from build123d import *

# Parameters (mm, degrees)
F0_W          = 812.8
F0_H          = 101.6
F1_DEPTH      = 482.6
F2_W          = 812.8
F2_H          = 228.6
F3_DEPTH      = 734.06
F3_DEPTH_BACK = 482.6
F4_W          = 812.8
F4_H          = 596.9
F5_DEPTH      = 1219.2
F6_W          = 812.8
F6_H          = 1397
F7_DEPTH      = 762
F8_W          = 657.52998
F8_H          = 629.62246
F9_DEPTH      = 774.7


with BuildPart() as f1:
    # F0 (on Top) → F1 (new body)
    with BuildSketch(Plane.XY):
        with Locations((406.4, 50.8)):
            Rectangle(F0_W, F0_H)
    extrude(amount=F1_DEPTH)

    # F2 (on face) → F3 (join, two sides)
    with BuildSketch(Plane.XY.offset(482.6)) as f3_sk:
        with Locations((406.4, 215.9)):
            Rectangle(F2_W, F2_H)
    extrude(amount=F3_DEPTH)
    extrude(f3_sk.sketch, amount=-F3_DEPTH_BACK)

    # F4 (on Top) → F5 (join)
    with BuildSketch(Plane.XY):
        with Locations((406.4, 628.65)):
            Rectangle(F4_W, F4_H)
    extrude(amount=F5_DEPTH)

    # F6 (on face) → F7 (join)
    with BuildSketch(Plane(origin=(0, 927.1, 0), x_dir=(-1, 0, 0), z_dir=(0, 1, 0))):
        with Locations((-406.4, 698.5)):
            Rectangle(F6_W, F6_H)
    extrude(amount=F7_DEPTH)

    # F8 (on face) → F9 (cut)
    with BuildSketch(Plane.XY.offset(1397)):
        with Locations((423.118338, 1320.792675)):
            Rectangle(F8_W, F8_H)
    extrude(amount=-F9_DEPTH, mode=Mode.SUBTRACT)


solid = f1.part
CAD build for the part. Positions are in the model's coordinates, mm. A direction names the side the tool comes from. Coordinates: 2 decimals unless noted, no trailing zeros. Loops run counter-clockwise (first coordinate to the right, second up) from the corner with the lowest first, then second, coordinate; pieces in that order, holes last. Notation, with made-up numbers: (80.5, -27.5) - (94.5, -27.5) arc R8 ccw to (94.5, -20.5) - close; hole circle Ø6 at (43, -14.75). An arc over 180 degrees is marked (long way). Use one line per item in the form item = value. Start each with the question number.
1) Band-saw the part on A-A (z = 872). Give the cut face in (x, y), and give its area (3 significant figures).
2) Drill centre lines: L1, parallel to X at y = 1047, z = 785; L2, parallel to Y at x = 287.5, z = 716; L3, parallel to Y at x = 432.5, z = 1288.5. Where is each one in solid material? Low to high. Write a range as from..to.
3) Band-saw the part on B-B (x = 318). Give the cut face in (y, z), and give its area (3 significant figures).
4) Tool access for faces 1 (the face through (419, 1005.981, 1015)), 2 (the face through (812.8, 833, 689)), 3 (the face through (401, 52, 482.6)): list every direction of +Z, -Z, +X, -X, +Y, -Y with a clear straight run to the whole face (end or side of a thin tool).
5) Flat gauge pins, fed straight in: pin 1 (2 mm diameter, centred on x = 215.5, z = 502.5, fed in from -Y); pin 2 (1.3 mm diameter, centred on x = 557.5, z = 1217.5, fed in from -Y). Where does each tip first touch, or does it go through?
6) Band-saw the part on C-C (y = 895). Give the cut face in (x, z), and give its area (3 significant figures).
7) Band-saw the part on D-D (y = 229). Give the cut face in (x, z), and give its area (3 significant figures).
8) Two-plate mould, pull along X, no slides. Class faces 4 (the face through (401, 101.6, 844)), 5 (the face through (0, 833, 689)), 6 (the face through (751.883, 1316, 1015)): +X half, -X half, draft (parallel to the pull), parting line (faces both ways), or undercut.
Check values:
q1.outline = (0, 101.6) - (812.8, 101.6) - (812.8, 1689.1) - (0, 1689.1) - close; hole (94.35, 1005.98) - (751.88, 1005.98) - (751.88, 1635.6) - (94.35, 1635.6) - close
q1.area = 876,000 mm2
q2.L1 = 0..94.35, 751.88..812.8
q2.L2 = 101.6..1005.98, 1635.6..1689.1
q2.L3 = 927.1..1005.98, 1635.6..1689.1
q3.outline = (0, 0) - (1689.1, 0) - (1689.1, 1397) - (1635.6, 1397) - (1635.6, 622.3) - (1005.98, 622.3) - (1005.98, 1397) - (927.1, 1397) - (927.1, 1219.2) - (330.2, 1219.2) - (330.2, 1216.66) - (101.6, 1216.66) - (101.6, 482.6) - (0, 482.6) - close
q3.area = 1,630,000 mm2
q4.face_1 = +Z
q4.face_2 = +Z, -Z, +X, +Y, -Y
q4.face_3 = +Z, +X, -X, -Y
q5.pin_1 = 101.6
q5.pin_2 = 330.2
q6.outline = (0, 0) - (812.8, 0) - (812.8, 1219.2) - (0, 1219.2) - close
q6.area = 991,000 mm2
q7.outline = (0, 0) - (812.8, 0) - (812.8, 1216.66) - (0, 1216.66) - close
q7.area = 989,000 mm2
q8.face_4 = draft
q8.face_5 = -X half
q8.face_6 = undercut
